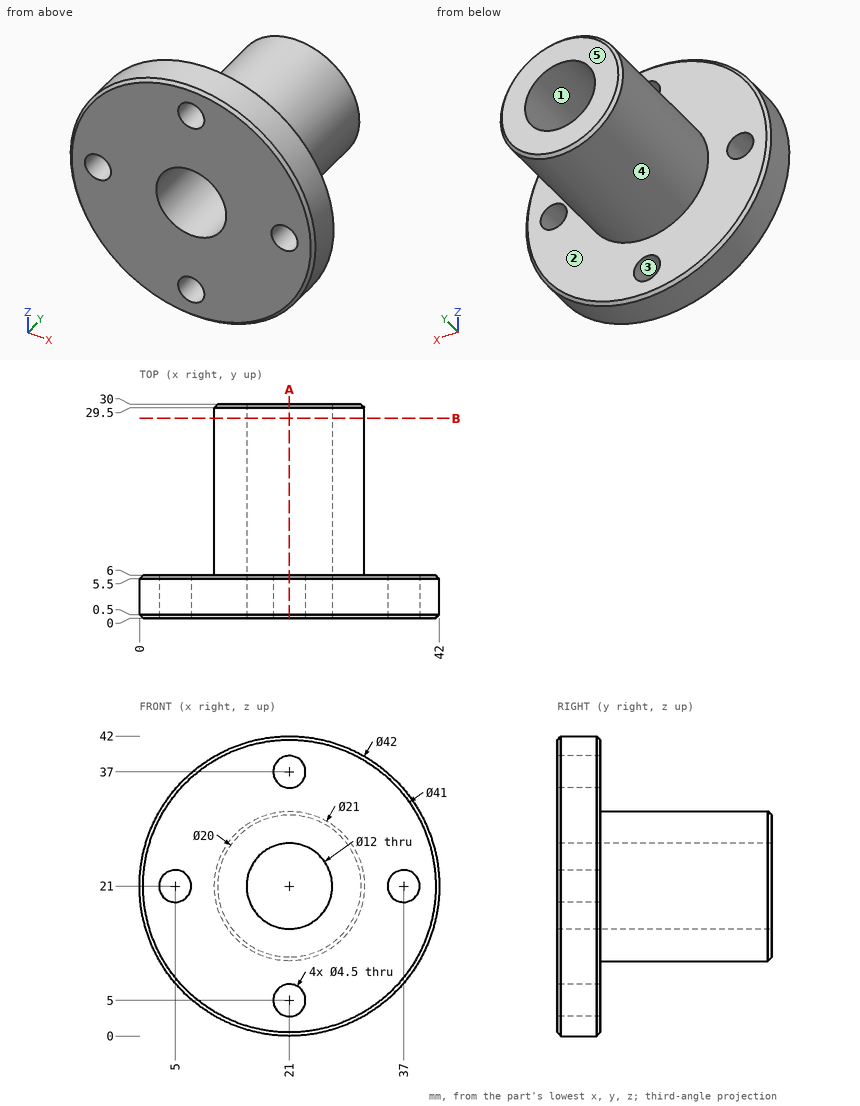
The drawing under review shows one solid part. Ordinate dimensions are in mm from its lowest x, y, z. A direction names the side the tool comes from. Round coordinates to 2 decimals unless told otherwise and drop trailing zeros. Order: outer loops, then holes, each group sorted by start corner. A loop starts at its lowest first (then second) coordinate and runs counter-clockwise, first axis right, second up. Notation, with made-up numbers: (85, 31.5) -> (93, 31.5) arc R29 cw to (93, 58.5) -> close; hole circle Ø1 at (40, -17). An arc over 180 degrees is marked (long way). Return JSON: item names as keys, results as strings.
1. For L1, parallel to X at y = 1.6, z = 21; L2, parallel to X at y = 10.75, z = 21; L3, parallel to Y at x = 29, z = 36, list the stretches that pass through material, from the lowest coordinate up. Write a range as [from, to].
Answer block:
{"L1": "x = [0, 2.75], [7.25, 15], [27, 34.75], [39.25, 42]", "L2": "x = [10.5, 15], [27, 31.5]", "L3": "y = [0, 6]"}
2. Take a section at B-B (y = 28). Write out the cut boundary in (x, z).
Answer block:
{"outline": "circle Ø21 at (21, 21); hole circle Ø12 at (21, 21)"}
3. Take a section at A-A (x = 21). Write out the cut boundary in (y, z).
Answer block:
{"outline": "(0, 0.5) -> (0.5, 0) -> (5.5, 0) -> (6, 0.5) -> (6, 2.75) -> (0, 2.75) -> close; (0, 7.25) -> (6, 7.25) -> (6, 10.5) -> (29.5, 10.5) -> (30, 11) -> (30, 15) -> (0, 15) -> close; (0, 27) -> (30, 27) -> (30, 31) -> (29.5, 31.5) -> (6, 31.5) -> (6, 34.75) -> (0, 34.75) -> close; (0, 39.25) -> (6, 39.25) -> (6, 41.5) -> (5.5, 42) -> (0.5, 42) -> (0, 41.5) -> close"}
4. For the marked faces 1 and 2, list the 3-axis set-ups (+Z, -Z, +X, -X, +Y, -Y) from which the entire face can be reached by the end or side of a thin tool; tool diameter is ignored.
Answer block:
{"face 1": "+Y, -Y", "face 2": "+Y"}
5. The part is to be moulded in two halves that separate along X. For the marked faces 3, 4 and 5, say which applies: +X half, -X half, draft (parallel to the pull), parting line (faces both ways), or undercut.
Answer block:
{"face 3": "undercut", "face 4": "parting line", "face 5": "draft"}
6. Insertion check: P1, Ø11, axis at x = 21, z = 21, coming from the -Y side; P2, Ø10, axis at x = 24.5, y = 17.5, coming from the -Z side; P3, Ø5, axis at x = 24.5, y = 26, coming from the +Z side; P4, Ø2, axis at x = 11.5, y = 3.5, coming from the +Z side. Each pin has a flat end and moves straight along its axis. Give the tip position at first contact, or say it passes through.
Answer block:
{"P1": "passes through", "P2": "stops at z = 10.5", "P3": "stops at z = 31.45", "P4": "stops at z = 40.2"}
